Read the model definition and answer for the solid it produces. Units are mm, in the model's axes. Face numbers are marked on the shaded views. Give positions to 0.01 mm unless a question says otherwise; leave off trailing zeros. Loops run counter-clockwise (first coordinate to the right, second up) from the corner with the lowest first, then second, coordinate; pieces in that order, holes last. Notation, with made-up numbers: (-2, -29.75) - (54, -29.75) arc R26 ccw to (54, -5.75) - close; hole circle Ø3 at (6.5, 85). An arc over 180 degrees is marked (long way). Put each result on its own line as item: value. Start each with the question number.
1. Consider L1, parallel to Y at x = 0.75, z = 1.3; L2, parallel to X at y = -7.5, z = 0.25; L3, parallel to X at y = 0.25, z = 1.65 (3 decimals). Determine where each line is inside the solid, lowest interval first. Write a range as from..to.
2. For a pull along X with two mould halves and no side action, classify the marked faces 1, 2 and 3 as released by +X, released by -X, zero draft, split by the parting line, or undercut.
3. A cutting plane is placed at C-C, the plane z = 0.3. Count the separate pieces of the cut face and the enclosed holes in it, plus the area to 3 significant figures.
4. A cutting plane is placed at A-A, the plane y = 0. Determine the outline of the cut face in (x, z) (3 decimals).
5. A cutting plane is placed at B-B, the plane x = 0.25. Determine the outline of the cut face in (y, z), plus the area to 3 significant figures.
6. A cutting plane is placed at D-D, the plane y = -3.25. Determine the outline of the cut face in (x, z) (3 decimals), plus the area to 3 significant figures.
7. Given pin 1 Ø1.2 at (x, y) = (1.875, -7) entering from +Z; pin 2 Ø1 at (x, z) = (-3, 2.5) entering from -Y, each flat-ended and moving along its own axis, determine where each tip first touches the part or whether it passes through.
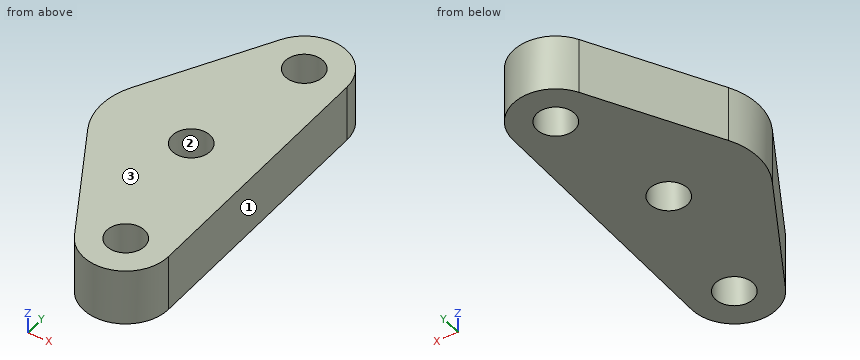
Autodesk Inventor part; units mm, degrees
ref_plane "YZ Plane" through (0, 0, 0) normal (1, 0, 0) x (0, 1, 0)
ref_plane "XZ Plane" through (0, 0, 0) normal (0, 1, 0) x (-1, 0, 0)
ref_plane "XY Plane" through (0, 0, 0) normal (0, 0, 1) x (1, 0, 0)
sketch "Sketch1" plane through (0, 0, 0) normal (0, 0, 1) x (1, 0, 0)
  line L0 (0.625, 2.5) -> (2.625, 2.5)
  line L1 (4.125, 1) -> (2.625, 2.5)
  line L2 (4.125, 7) -> (4.125, 1)
  arc A0 (4.125, 7) -> (-0.0865, 8.1023) centre (1.875, 7) ccw
  line L3 (-3.6762, 1.7147) -> (-0.0865, 8.1023)
  arc A1 (-3.6762, 1.7147) -> (-3.6762, -1.7147) centre (-0.625, 0) ccw
  line L4 (-0.0865, -8.1023) -> (-3.6762, -1.7147)
  arc A2 (-0.0865, -8.1023) -> (4.125, -7) centre (1.875, -7) ccw
  line L5 (4.125, -1) -> (4.125, -7)
  line L6 (2.625, -2.5) -> (4.125, -1)
  line L7 (2.625, -2.5) -> (0.625, -2.5)
  arc A3 (0.625, 2.5) -> (0.625, -2.5) centre (0.625, 0) ccw
  circle A4 centre (1.875, 7) radius 1
  circle A5 centre (1.875, -7) radius 1
  circle A6 centre (0.625, 0) radius 1
  line L8 (4.125, -1) -> (2.625, -2.5)
  line L9 (4.125, 1) -> (4.125, -1)
  line L10 (2.625, 2.5) -> (4.125, 1)
  line L11 (2.625, 2.5) -> (0.625, 2.5)
  arc A7 (0.625, 2.5) -> (0.625, -2.5) centre (0.625, 0) ccw
  line L12 (0.625, -2.5) -> (2.625, -2.5)
  point P0 (0, 0)
extrude "Extrusion1" add sketch "Sketch1" along normal blind 3
properties part number "belt_tender_2"
Return value:
1. L1: y = -8.95..-0.99, 0.99..8.95
1. L2: x = -0.42..1.01, 2.74..4.07
1. L3: x = -4.116..-0.343, 1.593..4.125
2. face 1: released by +X
2. face 2: undercut
2. face 3: zero draft
3. separate pieces: 1
3. enclosed holes: 3
3. area: 101 mm2
4. outline: (-4.125, 0) - (-0.375, 0) - (-0.375, 3) - (-4.125, 3) - close; (1.625, 0) - (4.125, 0) - (4.125, 3) - (1.625, 3) - close
5. outline: (-8.56, 0) - (-0.93, 0) - (-0.93, 3) - (-8.56, 3) - close; (0.93, 0) - (8.56, 0) - (8.56, 3) - (0.93, 3) - close
5. area: 45.8 mm2
6. outline: (-2.813, 0) - (4.125, 0) - (4.125, 3) - (-2.813, 3) - close
6. area: 20.8 mm2
7. pin 1: passes through
7. pin 2: stops at y = -3.81
